```python
from build123d import *

# Parameters (mm, degrees)
BOSS_EXTRUDE1_DEPTH = 3
SKETCH2_W           = 3
SKETCH2_H           = 10
CUT_EXTRUDE1_DEPTH  = 108.373181009
SKETCH3_R           = 4
CUT_EXTRUDE2_DEPTH  = 108.373181009
SKETCH4_W           = 3
SKETCH4_H           = 30
CUT_EXTRUDE3_DEPTH  = 108.373181009
CUT_EXTRUDE4_DEPTH  = 108.373181009


with BuildPart() as part:
    # Sketch1 → Boss-Extrude1 (new body)
    with BuildSketch(Plane.XY):
        Polygon((0, 0), (0, 96), (15.5, 96), (15.5, 93), (35.5, 93), (35.5, 96), (48, 96), (48, 0), (35.5, 0), (35.5, 3), (15.5, 3), (15.5, 0), align=None)
    extrude(amount=BOSS_EXTRUDE1_DEPTH)

    # Sketch2 → Cut-Extrude1 (cut, through all)
    with BuildSketch(Plane.XY.offset(3)):
        with Locations((1.5, 18)):
            Rectangle(SKETCH2_W, SKETCH2_H)
    extrude(amount=-CUT_EXTRUDE1_DEPTH, mode=Mode.SUBTRACT)

    # Sketch3 → Cut-Extrude2 (cut, through all)
    with BuildSketch(Plane(origin=(0, 0, 0), x_dir=(-1, 0, 0), z_dir=(0, 0, -1))):
        with Locations((-29, 48)):
            Circle(SKETCH3_R)
    extrude(amount=-CUT_EXTRUDE2_DEPTH, mode=Mode.SUBTRACT)

    # Sketch4 → Cut-Extrude3 (cut, through all)
    with BuildSketch(Plane(origin=(0, 0, 0), x_dir=(-1, 0, 0), z_dir=(0, 0, -1))):
        with Locations((-46.5, 48)):
            Rectangle(SKETCH4_W, SKETCH4_H)
    extrude(amount=-CUT_EXTRUDE3_DEPTH, mode=Mode.SUBTRACT)

    # Sketch5 → Cut-Extrude4 (cut, through all)
    with BuildSketch(Plane(origin=(0, 0, 0), x_dir=(-1, 0, 0), z_dir=(0, 0, -1))):
        with BuildLine():
            Line((-10, 57), (-30, 57))
            ThreePointArc((-30, 57), (-33.535533906, 58.464466094), (-35, 62))
            Line((-35, 62), (-35, 74))
            ThreePointArc((-35, 74), (-33.535533906, 77.535533906), (-30, 79))
            Line((-30, 79), (-10, 79))
            ThreePointArc((-10, 79), (-6.464466094, 77.535533906), (-5, 74))
            Line((-5, 74), (-5, 62))
            ThreePointArc((-5, 62), (-6.464466094, 58.464466094), (-10, 57))
        make_face()
    extrude(amount=-CUT_EXTRUDE4_DEPTH, mode=Mode.SUBTRACT)


solid = part.part
```
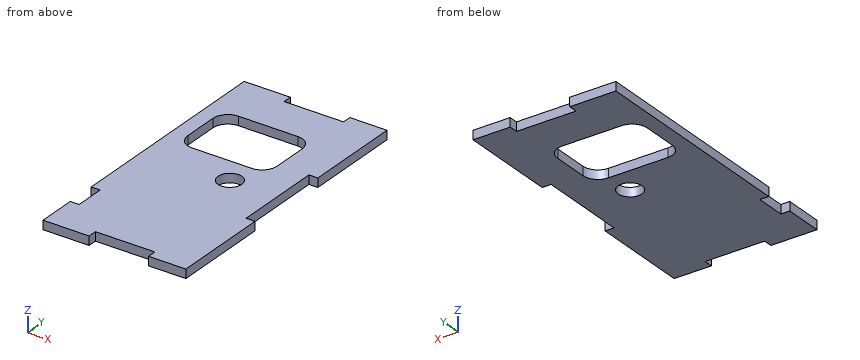
Design review of the part built by this model. Coordinates are the model's own, in mm. Coordinates: 2 decimals unless noted, no trailing zeros. Write each loop counter-clockwise with the first axis right and the second up, starting at its lowest first coordinate (ties: lowest second). Pieces come first, ordered by that corner, then holes. Notation, with made-up numbers: M 13.25,-22 L 62.25,-22 A18 ccw 62.25,-11 Z; hole C 88,-2 d1. An arc over 180 degrees is marked long. Answer as a JSON object with one key per item and string values.
Item 1: Add section D-D, the plane x = 7.5. Give the boundary of the cut face in (y, z), and give its area (3 significant figures).
Outcome:
{"outline": "M 0,0 L 57.67,0 L 57.67,3 L 0,3 Z; M 78.33,0 L 96,0 L 96,3 L 78.33,3 Z", "area": "226 mm²"}
Item 2: Wall thickness on probe 1 along Y at (x, z) = (29, 1.45); probe 2 along Y at (x, z) = (26, 1.8); probe 3 along Y at (x, z) = (12, 0.95): over which ranges is each line inside the solid? List them lowest first.
Outcome:
{"probe 1": "3 to 44, 52 to 57, 79 to 93", "probe 2": "3 to 45.35, 50.65 to 57, 79 to 93", "probe 3": "0 to 57, 79 to 96"}
Item 3: Add section A-A, the plane x = 29. Give the boundary of the cut face in (y, z).
Outcome:
{"outline": "M 3,0 L 44,0 L 44,3 L 3,3 Z; M 52,0 L 57,0 L 57,3 L 52,3 Z; M 79,0 L 93,0 L 93,3 L 79,3 Z"}
Item 4: Add section B-B, the plane y = 48. Give the boundary of the cut face in (x, z).
Outcome:
{"outline": "M 0,0 L 25,0 L 25,3 L 0,3 Z; M 33,0 L 45,0 L 45,3 L 33,3 Z"}
Item 5: Insertion check: pin 1 Ø0.9 at (y, z) = (95, 2) entering from -X; pin 2 Ø1.5 at (x, z) = (26.5, 1) entering from -Y; pin 3 Ø0.9 at (x, z) = (24.5, 1) entering from +Y; pin 4 Ø0.9 at (y, z) = (43, 1.5) entering from +X. Each pin has a flat end and moves straight along its axis. Give the tip position at first contact, or say it passes through.
Outcome:
{"pin 1": "x = 0", "pin 2": "y = 3", "pin 3": "y = 93", "pin 4": "x = 45"}
Item 6: Add section C-C, the plane z = 1.3. State how many separate pieces and enclosed holes the cut face has, and give its area (3 significant figures).
Outcome:
{"separate pieces": "1", "enclosed holes": "2", "area": "3,680 mm²"}
